Autodesk Inventor part; units mm, degrees
ref_plane "YZ Plane" through (0, 0, 0) normal (1, 0, 0) x (0, 1, 0)
ref_plane "XZ Plane" through (0, 0, 0) normal (0, 1, 0) x (-1, 0, 0)
ref_plane "XY Plane" through (0, 0, 0) normal (0, 0, 1) x (1, 0, 0)
sketch "Skizze1" plane through (0, 0, 0) normal (0, 0, 1) x (1, 0, 0)
  circle A0 centre (2.503632, -2.442355) radius 1.4 construction
  circle A1 centre (-2.548384, 2.392405) radius 1.4 construction
  arc A2 (8.895275, -1.548845) -> (-1.933457, 8.820314) centre (-14.431862, -15.070948) ccw
  line L0 (-1.933457, 8.820314) -> (-8.895275, 1.545658)
  line L1 (-8.895275, 1.545658) -> (1.936506, -8.820314)
  line L2 (1.936506, -8.820314) -> (8.895275, -1.548845)
  arc A3 (-17.414954, -14.752893) -> (-12.725508, -17.538408) centre (-14.431862, -15.070948) ccw
  line L3 (-8.895275, 1.545658) -> (-25.488913, -15.793637)
  line L4 (-25.488913, -15.793637) -> (-14.657133, -26.159609)
  line L5 (-14.657133, -26.159609) -> (1.936506, -8.820314)
  arc A4 (-13.288846, -12.847547) -> (-12.20846, -16.213964) centre (-14.431862, -15.070948) ccw
  circle A5 centre (-14.431862, -15.070948) radius 3.1
  circle A6 centre (-2.548384, 2.392405) radius 1.6
  circle A7 centre (2.503632, -2.442355) radius 1.6
  circle A8 centre (-22.802017, -23.070943) radius 1.4
  circle A9 centre (-6.057441, -7.070954) radius 1.4
  point P0 (0, 0)
  dimension "d0" = 24
  dimension "d1" = 6.2
  dimension "d2" = 3.2
  dimension "d3" = 3.2
extrude "Extrusion1" add sketch "Skizze1" along normal blind 15 contours L2 L1 L0 A2 | L5 L4 L3 L1 | A9
sketch "Skizze2" plane through (0, 0, 15) normal (0, 0, 1) x (1, 0, 0)
  point P0 (0, 0)
sketch "Skizze3" plane through (0, 0, 15) normal (0, 0, 1) x (1, 0, 0)
  point P0 (0, 0)
fillet "Rundung1" radius 2 2 edges at (-14.6571, -26.1596, 7.5) (-25.4889, -15.7936, 7.5)
sketch "Skizze4" plane through (0, 0, 0) normal (0, 0, -1) x (-1, 0, 0)
  circle A0 centre (14.431862, -15.070948) radius 3.1
  line L0 (21.161771, -13.42525) -> (19.222032, -20.076372)
  line L1 (19.222032, -20.076372) -> (12.492123, -21.72207)
  line L2 (12.492123, -21.72207) -> (7.701952, -16.716646)
  line L3 (7.701952, -16.716646) -> (9.641691, -10.065525)
  line L4 (9.641691, -10.065525) -> (16.3716, -8.419827)
  line L5 (16.3716, -8.419827) -> (21.161771, -13.42525)
  line L6 (1.933457, 8.820314) -> (24.10611, -14.348696)
  point P0 (0, 0)
  dimension "d10" = 12
sketch "Skizze4 outline for Extrusion2" plane through (0, 0, 0) normal (0, 0, -1) x (-1, 0, 0)
  line L0 (21.161771, -13.42525) -> (16.3716, -8.419827)
  line L1 (19.222032, -20.076372) -> (21.161771, -13.42525)
  line L2 (12.492123, -21.72207) -> (19.222032, -20.076372)
  line L3 (7.701952, -16.716646) -> (12.492123, -21.72207)
  line L4 (9.641691, -10.065525) -> (7.701952, -16.716646)
  line L5 (16.3716, -8.419827) -> (9.641691, -10.065525)
extrude "Extrusion2" cut sketch "Skizze4 outline for Extrusion2" against normal blind 5 draft -2
properties part number "IM_Matchboxscope_Laserholder_M12"
Here's how the part is built. I have some questions about the finished solid (model axes, mm). A direction names the side the tool comes from. Give positions to 0.01 mm unless a question says otherwise; leave off trailing zeros. Order: outer loops, then holes, each group sorted by start corner. A loop starts at its lowest first (then second) coordinate and runs counter-clockwise, first axis right, second up. Notation, with made-up numbers: (62.5, 5.5) -> (79.5, 5.5) arc R26 ccw to (79.5, 41.5) -> close; hole circle Ø9 at (65, 44). An arc over 180 degrees is marked (long way). One line per item, written item: value. Start each with the question number.
1. Imagine slicing it at C-C, the plane y = -11. List the corners of the cut face in (x, z) for me.
2. Imagine slicing it at A-A, the plane x = -12. List the corners of the cut face in (y, z) for me.
3. Will these pins go through, and if not, where does the flat tip stop? pin 1 Ø8 at (y, z) = (-13.5, 4) entering from +X; pin 2 Ø8 at (x, z) = (-5.5, 2.5) entering from +Y; pin 3 Ø3 at (y, z) = (-20, 10) entering from +X.
4. Imagine slicing it at B-B, the plane z = 1. List the corners of the cut face in (x, y) for me, plus the area to 3 significant figures.
5. We'd pull the mould along X, two halves only. Please class faces 3 (the face through (-24.66, -15.75, 7.6)), 4 (the face through (-14.7, -25.33, 7.6)), 5 (the face through (-3.728, 1.311, 7.395)): released by +X, released by -X, zero draft, split by the parting line, or undercut.
6. Imagine slicing it at D-D, the plane z = 14. List the corners of the cut face in (x, y) for me, plus the area to 3 significant figures.
7. For faces 1 (the face through (-5, -7, 0)), 2 (the face through (-13, -18, 5)), which set-ups out of +Z, -Z, +X, -X, +Y, -Y let a thin tool reach every point of the face, with its end or its side?
8. I need wall thicknesses on probe 1 along Y at (x, z) = (-4, 4.25); probe 2 along Y at (x, z) = (-3.5, 9.5); probe 3 along X at (y, z) = (-3, 9.5). Which ranges of each line are inside material? Lowest first, please. Write a range as from..to.
Values follow:
1. outline: (-20.9, 0) -> (-18.84, 0) -> (-18.6, 5) -> (-9.55, 5) -> (-9.37, 0) -> (-0.15, 0) -> (-0.15, 15) -> (-20.9, 15) -> close
2. outline: (-23.38, 0) -> (-21.21, 0) -> (-20.96, 5) -> (-16.99, 5) -> (-16.99, 15) -> (-23.38, 15) -> close; (-13.15, 5) -> (-9.67, 5) -> (-9.49, 0) -> (-1.7, 0) -> (-1.7, 15) -> (-13.15, 15) -> close
3. pin 1: stops at x = 1.29
3. pin 2: stops at y = 8.82
3. pin 3: stops at x = -7.33
4. outline: (-24.11, -14.35) arc R2 ccw to (-24.04, -17.18) -> (-16.1, -24.78) arc R2 ccw to (-13.27, -24.71) -> (8.9, -1.55) arc R26.96 ccw to (-1.93, 8.82) -> close; hole (-21.12, -13.43) -> (-19.19, -20.05) -> (-12.5, -21.68) -> (-7.74, -16.71) -> (-9.67, -10.09) -> (-16.36, -8.46) -> close; hole circle Ø3.2 at (-2.55, 2.39); hole circle Ø3.2 at (2.5, -2.44)
4. area: 380 mm2
5. face 3: released by -X
5. face 4: split by the parting line
5. face 5: undercut
6. outline: (-24.11, -14.35) arc R2 ccw to (-24.04, -17.18) -> (-16.1, -24.78) arc R2 ccw to (-13.27, -24.71) -> (8.9, -1.55) arc R26.96 ccw to (-1.93, 8.82) -> close; hole circle Ø6.2 at (-14.43, -15.07); hole circle Ø3.2 at (-2.55, 2.39); hole circle Ø3.2 at (2.5, -2.44)
6. area: 473 mm2
7. face 1: -Z, +X, -X, +Y, -Y
7. face 2: -Z
8. probe 1: y = -15.02..1.72, 3.07..6.66
8. probe 2: y = -14.5..1.11, 3.68..7.18
8. probe 3: x = -13.25..1, 4..7.51
